Read the model definition and answer for the solid it produces. Units are mm, in the model's axes. Give positions to 0.01 mm unless a question says otherwise; leave off trailing zeros. Order: outer loops, then holes, each group sorted by start corner. A loop starts at its lowest first (then second) coordinate and runs counter-clockwise, first axis right, second up. Notation, with made-up numbers: (33.5, 16) - (70.5, 16) arc R12 ccw to (70.5, 37) - close; hole circle Ø2 at (75, 4.25). An arc over 180 degrees is marked (long way). Write item = value, one per line.
```python
from build123d import *

# Parameters (mm, degrees)
F0_R     = 8.25
F0_R_2   = 4.5
F1_DEPTH = 4.1
F2_SIZE2 = 0.49999
F2_SIZE  = 4.09999
F3_R     = 1


# Not quite as in the source:
# - a fillet or chamfer is up to 0.001 mm smaller than in the source, because OpenCascade refuses the exact size


with BuildPart() as f1:
    # F0 (on Top) → F1 (new body)
    with BuildSketch(Plane.XY):
        Circle(F0_R)
        Circle(F0_R_2, mode=Mode.SUBTRACT)
    extrude(amount=F1_DEPTH)

    # F2 (size 4.1 and 0.5 in the source; OpenCascade refuses exactly that, so slightly less here)
    f2_edges = [f1.edges().sort_by_distance(p)[0] for p in [
        (-4.5, 0, 4.1),
    ]]
    f2_side = f1.faces().sort_by_distance((-4.5, 0, 2.05))[0]
    chamfer(f2_edges, length=F2_SIZE, length2=F2_SIZE2, reference=f2_side)

    # F3
    f3_edges = [f1.edges().sort_by_distance(p)[0] for p in [
        (-8.25, 0, 4.1),
    ]]
    fillet(f3_edges, radius=F3_R)


solid = f1.part
```
1. Determine the mould class of faces 1 (the face through (7.62, -3.16, 1.53)), 2 (the face through (-2, -5, 4.1)), 3 (the face through (2.168, -4.168, 1.623)) for opening direction Y: +Y half, -Y half, draft (parallel to the pull), parting line (faces both ways), or undercut.
Recorded:
face_1 = parting line
face_2 = draft
face_3 = undercut
2. Section C-C (z = 0.3) is taken. Determine the outline of the cut face in (x, y).
Recorded:
outline = circle Ø16.5 at (0, 0); hole circle Ø9.07 at (0, 0)
3. A flat-ended cylindrical pin translates along its axis: pin 1 (1 mm diameter, centred on y = 1.5, z = 2, fed in from +X). Find the tip coordinate at first contact, or state that the pin passes through.
Recorded:
pin_1 = 8.19
4. Section D-D (z = 2.3) is taken. Determine the outline of the cut face in (x, y).
Recorded:
outline = circle Ø16.5 at (0, 0); hole circle Ø9.56 at (0, 0)
5. Straight lines are drawn through the part: L1, parallel to Y at x = 0, z = 0.05; L2, parallel to Y at x = 3.5, z = 1.35; L3, parallel to X at y = 2.5, z = 1.5. For each, find the intervals that lie inside material, in ascending order. Write a range as [from, to].
Recorded:
L1 = [-8.25, -4.51], [4.51, 8.25]
L2 = [-7.47, -3.08], [3.08, 7.47]
L3 = [-7.86, -3.96], [3.96, 7.86]
